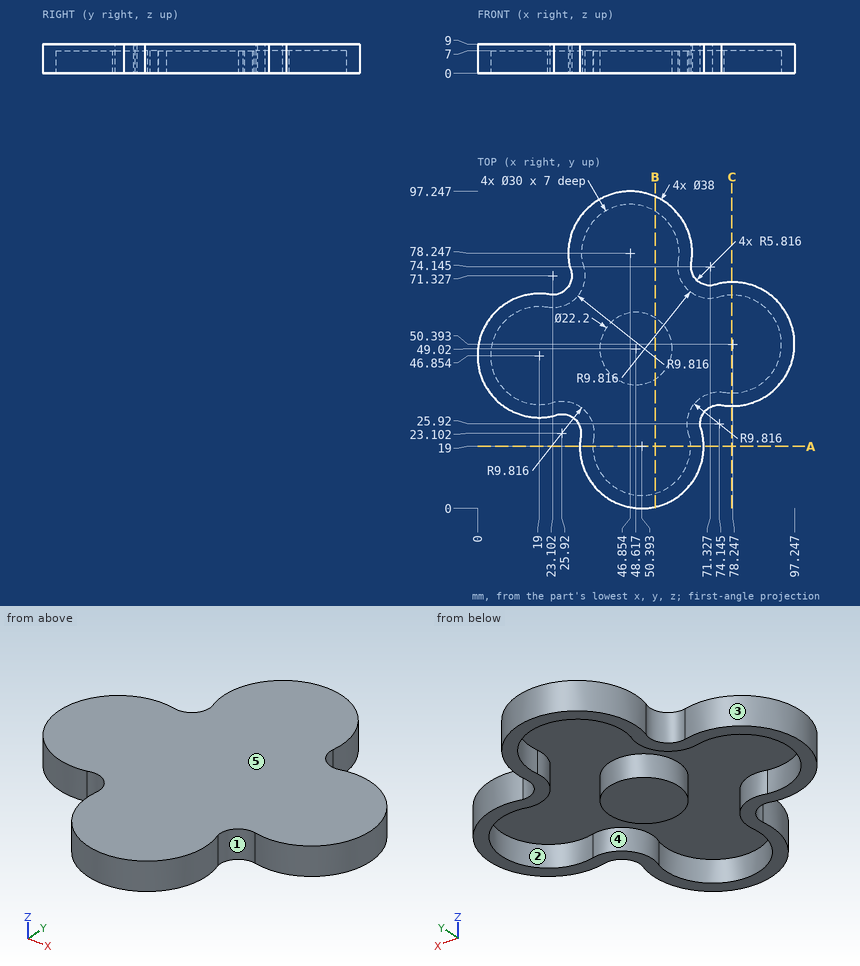
Geometry: see drawing. Coordinates: mm, zero at the bounding-box minimum. A direction names the side the tool comes from. Give positions to 0.01 mm unless a question says otherwise; leave off trailing zeros. Write each loop counter-clockwise with the first axis right and the second up, starting at its lowest first coordinate (ties: lowest second). Pieces come first, ordered by that corner, then holes. Notation, with made-up numbers: (-24.5, 22) -> (32.5, 22) arc R34 cw to (32.5, 52) -> close; hole circle Ø6 at (10.5, 86.25). An arc over 180 degrees is marked (long way). Use one line per item in the form item = value. Start each with the question number.
1) Section query C-C on x = 78. Return the cut outline in (y, z) (1 decimal).
2) Set-up query: the marked faces 1 and 2. Return all of +Z, -Z, +X, -X, +Y, -Y with unobstructed straight access to the full face (end or side cutting, diameter ignored); none if empty.
3) Ray query, probe 1 along Y at (x, z) = (19, 5.25) (1 decimal); probe 2 along X at (y, z) = (19, 2.75); probe 3 along Y at (x, z) = (20.5, 4.25) (1 decimal). Return the intervals inside material, ascending. Write a range as from..to.
4) Section query A-A on y = 19. Return the cut outline in (x, z).
5) Pin query (flat end, axial travel): pin 1 (1.5 mm diameter, centred on y = 31.5, z = 4.5, fed in from -X) (1 decimal); pin 2 (1 mm diameter, centred on x = 46.5, z = 8, fed in from +Y); pin 3 (4 mm diameter, centred on x = 26.5, y = 54.5, fed in from -Z); pin 4 (4 mm diameter, centred on x = 72.5, z = 1.5, fed in from +Y). Return the tip coordinate at first contact, or that it passes through.
6) Section query B-B on x = 54.5. Return the cut outline in (y, z).
7) Draft query along Y for the marked faces 3, 4 and 5. Return one class per face: pulls with the +Y half, pulls with the -Y half, needs draft (parallel to the pull), parting line crosses it, or undercut.
Outcome:
q1.outline = (31.4, 0) -> (35.4, 0) -> (35.4, 7) -> (65.4, 7) -> (65.4, 0) -> (69.4, 0) -> (69.4, 9) -> (31.4, 9) -> close
q2.face_1 = +Z, -Z
q2.face_2 = -Z
q3.probe_1 = 27.9..31.9, 61.9..65.9
q3.probe_2 = 31.39..35.39, 65.39..69.39
q3.probe_3 = 27.9..31.9, 61.8..65.8
q4.outline = (31.39, 0) -> (35.39, 0) -> (35.39, 7) -> (65.39, 7) -> (65.39, 0) -> (69.39, 0) -> (69.39, 9) -> (31.39, 9) -> close
q5.pin_1 = 6.8
q5.pin_2 = 97.25
q5.pin_3 = 7
q5.pin_4 = 69.02
q6.outline = (0.45, 0) -> (4.57, 0) -> (4.57, 7) -> (39.61, 7) -> (39.61, 0) -> (58.43, 0) -> (58.43, 7) -> (91.15, 7) -> (91.15, 0) -> (95.64, 0) -> (95.64, 9) -> (0.45, 9) -> close
q7.face_3 = parting line crosses it
q7.face_4 = undercut
q7.face_5 = needs draft
